Design review of the part built by this model. Coordinates are the model's own, in mm. Coordinates: 2 decimals unless noted, no trailing zeros. Answer as a JSON object with one key per item and string values.
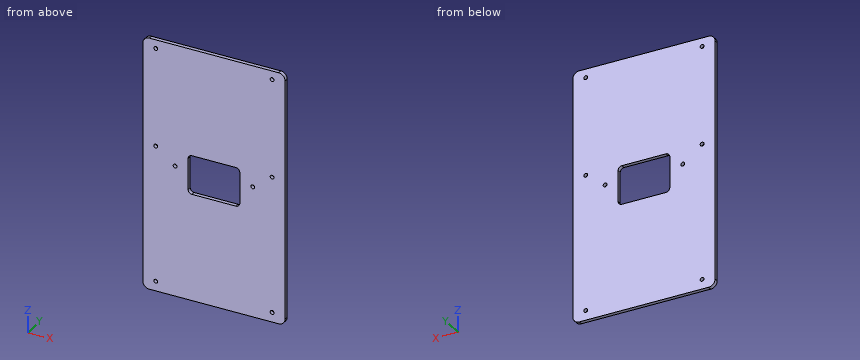
from build123d import *

# Parameters (mm, degrees)
CROQUIS1_W              = 110
CROQUIS1_H              = 195
SALIENTE_EXTRUIR1_DEPTH = 3
REDONDEO1_R             = 5
CROQUIS2_R              = 1.5
CORTAR_EXTRUIR1_DEPTH   = 3
CROQUIS3_W              = 40
CROQUIS3_H              = 30
CORTAR_EXTRUIR2_DEPTH   = 3
REDONDEO2_R             = 3


with BuildPart() as part:
    # Croquis1 → Saliente-Extruir1 (new body)
    with BuildSketch(Plane(origin=(0, 0, 0), x_dir=(1, 0, 0), z_dir=(0, 1, 0))):
        Rectangle(CROQUIS1_W, CROQUIS1_H)
    extrude(amount=SALIENTE_EXTRUIR1_DEPTH)

    # Redondeo1
    redondeo1_edges = [part.edges().sort_by_distance(p)[0] for p in [
        (55, 1.5, 97.5),
        (-55, 1.5, 97.5),
        (-55, 1.5, -97.5),
        (55, 1.5, -97.5),
    ]]
    fillet(redondeo1_edges, radius=REDONDEO1_R)

    # Croquis2 → Cortar-Extruir1 (cut)
    with BuildSketch(Plane(origin=(0, 3, 0), x_dir=(1, 0, 0), z_dir=(0, 1, 0))):
        with Locations(Location((-45, -90.857864376, 0), (0, 0, 270))):
            Circle(CROQUIS2_R)
        with Locations(Location((-45, -15, 0), (0, 0, 270))):
            Circle(CROQUIS2_R)
        with Locations(Location((-45, 90, 0), (0, 0, 270))):
            Circle(CROQUIS2_R)
        with Locations(Location((45, 90, 0), (0, 0, 270))):
            Circle(CROQUIS2_R)
        with Locations(Location((45, -15, 0), (0, 0, 270))):
            Circle(CROQUIS2_R)
        with Locations(Location((45, -90.857864376, 0), (0, 0, 270))):
            Circle(CROQUIS2_R)
        with Locations(Location((-30, -3.5, 0), (0, 0, 270))):
            Circle(CROQUIS2_R)
        with Locations(Location((30, -3.5, 0), (0, 0, 270))):
            Circle(CROQUIS2_R)
    extrude(amount=-CORTAR_EXTRUIR1_DEPTH, mode=Mode.SUBTRACT)

    # Croquis3 → Cortar-Extruir2 (cut)
    with BuildSketch(Plane(origin=(0, 3, 0), x_dir=(1, 0, 0), z_dir=(0, 1, 0))):
        Rectangle(CROQUIS3_W, CROQUIS3_H)
    extrude(amount=-CORTAR_EXTRUIR2_DEPTH, mode=Mode.SUBTRACT)

    # Redondeo2
    redondeo2_edges = [part.edges().sort_by_distance(p)[0] for p in [
        (20, 1.5, -15),
        (20, 1.5, 15),
        (-20, 1.5, 15),
        (-20, 1.5, -15),
    ]]
    fillet(redondeo2_edges, radius=REDONDEO2_R)


solid = part.part
1) To check wall thickness, follow L1, parallel to X at y = 1.6, z = -90; L2, parallel to X at y = 2, z = 3.5; L3, parallel to Z at x = -12, y = 1.8. State the ranges of each line that lie inside material, in increasing order.
Taken from the geometry:
{"L1": "x = -55 to -46.5, -43.5 to 43.5, 46.5 to 55", "L2": "x = -55 to -31.5, -28.5 to -20, 20 to 28.5, 31.5 to 55", "L3": "z = -97.5 to -15, 15 to 97.5"}
2) Insertion check: pin 1 Ø2.5 at (x, z) = (45, -90) entering from +Y. The pin has a flat end and moves straight along its axis. Give the tip position at first contact, or say it passes through.
Taken from the geometry:
{"pin 1": "passes through"}
3) Add section A-A (y = 0.65). Count the separate pieces of the cut face and the enclosed holes in it, and give its area (3 significant figures).
Taken from the geometry:
{"separate pieces": "1", "enclosed holes": "9", "area": "20,200 mm2"}
